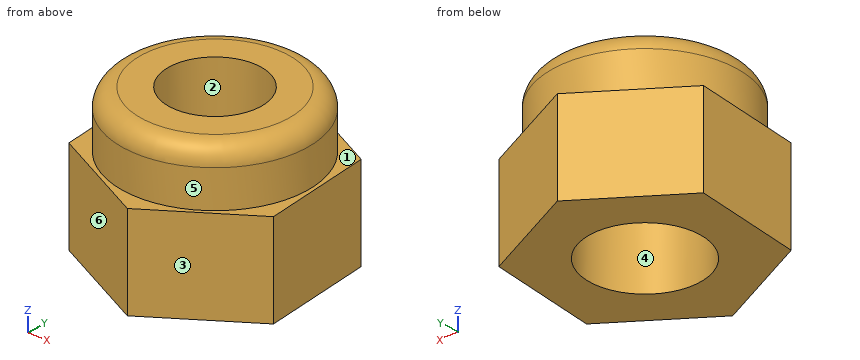
```python
from build123d import *

# Parameters (mm, degrees)
SKETCH_1_R      = 2.5
SKETCH_1_R_2    = 1.25
EXTRUDE_1_DEPTH = 1.5
FILLET_1_R      = 0.5
SKETCH_2_R      = 1.5
EXTRUDE_2_DEPTH = 2.5


with BuildPart() as part:
    # 草图1 → 凸台-拉伸1 (new body)
    with BuildSketch(Plane.XY):
        Circle(SKETCH_1_R)
        Circle(SKETCH_1_R_2, mode=Mode.SUBTRACT)
    extrude(amount=EXTRUDE_1_DEPTH)

    # 圆角1
    fillet_1_edges = [part.edges().sort_by_distance(p)[0] for p in [
        (-2.5, 0, 1.5),
    ]]
    fillet(fillet_1_edges, radius=FILLET_1_R)

    # 草图2 → 凸台-拉伸2 (add)
    with BuildSketch(Plane(origin=(0, 0, 0), x_dir=(-1, 0, 0), z_dir=(0, 0, -1))):
        Polygon((2.433288981, -1.748657981), (2.731026725, 1.232961082), (0.297737744, 2.981619063), (-2.433288981, 1.748657981), (-2.731026725, -1.232961082), (-0.297737744, -2.981619063), align=None)
        Circle(SKETCH_2_R, mode=Mode.SUBTRACT)
    extrude(amount=EXTRUDE_2_DEPTH)


solid = part.part
```
The listing builds one solid part. Answer for the finished solid, in the listing's coordinates (mm). Face numbers are marked on the shaded views. A direction names the side the tool comes from. Give positions to 0.01 mm unless a question says otherwise; leave off trailing zeros. Loops run counter-clockwise (first coordinate to the right, second up) from the corner with the lowest first, then second, coordinate; pieces in that order, holes last. Notation, with made-up numbers: (8, 18.25) - (26, 18.25) arc R25 ccw to (26, 42.25) - close; hole circle Ø1 at (77.5, -8.75). An arc over 180 degrees is marked (long way). Answer as CSV lines item,"result". Start each with the question number.
Item 1: A cutting plane is placed at D-D on z = 0.25. Determine the outline of the cut face in (x, y), then the cut area to 3 significant figures.
Item 2: Find the intervals of material crossed by line 1 (Y direction, x = 0, z = 0.35); line 2 (X direction, y = -0.85, z = 0.7); line 3 (X direction, y = -0.8, z = -1.75), in increasing order. Write a range as from..to.
Item 3: The mould has two halves that part along X. Classify the marked faces 1, 2, 3 and 4: +X half, -X half, draft (parallel to the pull), parting line (faces both ways), or undercut.
Item 4: For the marked faces 5 and 6, determine the directions among +Z, -Z, +X, -X, +Y, -Y from which every point of the face is accessible in a straight line to the end or side of a thin tool.
Item 5: A cutting plane is placed at C-C on y = 0. Determine the outline of the cut face in (x, z), then the cut area to 3 significant figures.
Item 6: This flat-tipped pin is pushed along its axis until it touches: pin 1 (1.5 mm diameter, centred on x = -2, y = -1, fed in from +Z). Where does it stop, or does it pass through?
Item 7: A cutting plane is placed at B-B on x = 0. Determine the outline of the cut face in (y, z).
Item 8: A cutting plane is placed at A-A on z = -1.85. Determine the outline of the cut face in (x, y).
Found:
1,outline,"circle Ø5 at (0, 0); hole circle Ø2.5 at (0, 0)"
1,area,"14.7 mm^2"
2,line 1,"y = -2.5..-1.25, 1.25..2.5"
2,line 2,"x = -2.35..-0.92, 0.92..2.35"
2,line 3,"x = -2.53..-1.27, 1.27..2.69"
3,face 1,"draft"
3,face 2,"undercut"
3,face 3,"+X half"
3,face 4,"undercut"
4,face 5,"+Z"
4,face 6,"+Z, -Z, -X, -Y"
5,outline,"(-2.61, -2.5) - (-1.5, -2.5) - (-1.5, 0) - (-1.25, 0) - (-1.25, 1.5) - (-2, 1.5) arc R0.5 ccw to (-2.5, 1) - (-2.5, 0) - (-2.61, 0) - close; (1.25, 0) - (1.5, 0) - (1.5, -2.5) - (2.61, -2.5) - (2.61, 0) - (2.5, 0) - (2.5, 1) arc R0.5 ccw to (2, 1.5) - (1.25, 1.5) - close"
5,area,"9.18 mm^2"
6,pin 1,"stops at z = 1.5"
7,outline,"(-2.85, -2.5) - (-1.5, -2.5) - (-1.5, 0) - (-1.25, 0) - (-1.25, 1.5) - (-2, 1.5) arc R0.5 ccw to (-2.5, 1) - (-2.5, 0) - (-2.85, 0) - close; (1.25, 0) - (1.5, 0) - (1.5, -2.5) - (2.85, -2.5) - (2.85, 0) - (2.5, 0) - (2.5, 1) arc R0.5 ccw to (2, 1.5) - (1.25, 1.5) - close"
8,outline,"(-2.73, 1.23) - (-2.43, -1.75) - (0.3, -2.98) - (2.73, -1.23) - (2.43, 1.75) - (-0.3, 2.98) - close; hole circle Ø3 at (0, 0)"
